Could you check a few things on this model? Use its own coordinates, in mm. A direction names the side the tool comes from. Give positions to 0.01 mm unless a question says otherwise; leave off trailing zeros. Order: outer loops, then holes, each group sorted by start corner. A loop starts at its lowest first (then second) coordinate and runs counter-clockwise, first axis right, second up. Notation, with made-up numbers: (4, 86.25) -> (34, 86.25) arc R13 cw to (34, 111.25) -> close; hole circle Ø7 at (25.25, 15). An arc over 180 degrees is marked (long way). Write each question's results on one line, items separated by ' | '.
```python
from build123d import *

# Parameters (mm, degrees)
SKETCH1_R           = 14
BOSS_EXTRUDE1_DEPTH = 20
SKETCH3_R           = 4.5
BOSS_EXTRUDE2_DEPTH = 1.5
SKETCH4_R           = 2.5
BOSS_EXTRUDE3_DEPTH = 8.5
CUT_EXTRUDE1_DEPTH  = 6


with BuildPart() as part:
    # Sketch1 → Boss-Extrude1 (new body)
    with BuildSketch(Plane(origin=(0, 0, 0), x_dir=(1, 0, 0), z_dir=(0, 1, 0))):
        Circle(SKETCH1_R)
    extrude(amount=BOSS_EXTRUDE1_DEPTH)

    # Sketch3 → Boss-Extrude2 (add)
    with BuildSketch(Plane(origin=(0, 20, 0), x_dir=(1, 0, 0), z_dir=(0, 1, 0))):
        with Locations((0, 8)):
            Circle(SKETCH3_R)
    extrude(amount=BOSS_EXTRUDE2_DEPTH)

    # Sketch4 → Boss-Extrude3 (add)
    with BuildSketch(Plane(origin=(0, 21.5, 0), x_dir=(1, 0, 0), z_dir=(0, 1, 0))):
        with Locations((0, 8)):
            Circle(SKETCH4_R)
    extrude(amount=BOSS_EXTRUDE3_DEPTH)

    # Sketch5 → Cut-Extrude1 (cut)
    with BuildSketch(Plane(origin=(0, 30, 0), x_dir=(1, 0, 0), z_dir=(0, 1, 0))):
        with BuildLine():
            Line((2, 9.5), (-2, 9.5))
            ThreePointArc((-2, 9.5), (0, 10.5), (2, 9.5))
        make_face()
        with BuildLine():
            Line((-2, 6.5), (2, 6.5))
            ThreePointArc((2, 6.5), (0, 5.5), (-2, 6.5))
        make_face()
    extrude(amount=-CUT_EXTRUDE1_DEPTH, mode=Mode.SUBTRACT)


solid = part.part
```
Q1. I'm going to push flat-ended pins straight in: pin 1 Ø2 at (y, z) = (5.5, 3.5) entering from -X (3 decimals); pin 2 Ø3 at (x, z) = (-1.5, -5.5) entering from +Y; pin 3 Ø6 at (x, y) = (-11, 11) entering from -Z; pin 4 Ø1.5 at (x, y) = (-8, 8.5) entering from +Z. Where does each tip first touch, or does it pass through?
Here are the results:
pin 1: stops at x = -13.775 | pin 2: stops at y = 30 | pin 3: stops at z = -11.49 | pin 4: stops at z = 11.98
Q2. I need wall thicknesses on line 1 along Y through (x, z) = (-12.75, 3); line 2 along Z through (x, y) = (0.5, 1.5); line 3 along X through (y, z) = (9, -4). Which ranges of each line are inside material? Lowest first, please.
Here are the results:
line 1: y = 0 to 20 | line 2: z = -13.99 to 13.99 | line 3: x = -13.42 to 13.42
Q3. For faces 1 (the cylindrical face through (-0.59, 20.74, -12.46)), 2 (the flat face through (0, 27, -6.5)), 3 (the flat face through (0, 27, -9.5)), which set-ups out of +Z, -Z, +X, -X, +Y, -Y let a thin tool reach every point of the face, with its end or its side?
Here are the results:
face 1: +Y | face 2: +Z, +X, -X, +Y | face 3: -Z, +X, -X, +Y
Q4. Suppose I cut it at C-C on y = 13.5. Please give me the cut outline in (x, z).
Here are the results:
outline: circle Ø28 at (0, 0)
Q5. Suppose I cut it at D-D on z = -8. Please give me the cut outline in (x, y).
Here are the results:
outline: (-11.49, 0) -> (11.49, 0) -> (11.49, 20) -> (4.5, 20) -> (4.5, 21.5) -> (2.5, 21.5) -> (2.5, 30) -> (-2.5, 30) -> (-2.5, 21.5) -> (-4.5, 21.5) -> (-4.5, 20) -> (-11.49, 20) -> close
Q6. Suppose I cut it at A-A on x = 0. Please give me the cut outline in (y, z), and give its area (3 significant figures).
Here are the results:
outline: (0, -14) -> (20, -14) -> (20, -12.5) -> (21.5, -12.5) -> (21.5, -10.5) -> (24, -10.5) -> (24, -9.5) -> (30, -9.5) -> (30, -6.5) -> (24, -6.5) -> (24, -5.5) -> (21.5, -5.5) -> (21.5, -3.5) -> (20, -3.5) -> (20, 14) -> (0, 14) -> close | area: 604 mm²
Q7. Suppose I cut it at B-B on z = -4.75. Please give me the cut outline in (x, y), and give its area (3 significant figures).
Here are the results:
outline: (-13.17, 0) -> (13.17, 0) -> (13.17, 20) -> (3.11, 20) -> (3.11, 21.5) -> (-3.11, 21.5) -> (-3.11, 20) -> (-13.17, 20) -> close | area: 536 mm²
